Work out the finished part from the listing and answer in its coordinate system (mm). A direction names the side the tool comes from. Coordinates: 2 decimals unless noted, no trailing zeros. Order: outer loops, then holes, each group sorted by start corner. A loop starts at its lowest first (then second) coordinate and runs counter-clockwise, first axis right, second up. Notation, with made-up numbers: (51.5, 78.25) -> (101.5, 78.25) arc R29 ccw to (101.5, 108.25) -> close; hole circle Ø6 at (80, 86.25). An arc over 180 degrees is marked (long way). Use one line per item in the form item = value.
from build123d import *

# Parameters (mm, degrees)
SKETCH1_W           = 1000
SKETCH1_H           = 1000
BOSS_EXTRUDE1_DEPTH = 10
SKETCH2_R           = 150
BOSS_EXTRUDE2_DEPTH = 300
SKETCH3_R           = 25
CUT_EXTRUDE1_DEPTH  = 50


with BuildPart() as part:
    # Sketch1 → Boss-Extrude1 (new body)
    with BuildSketch(Plane(origin=(0, 0, 0), x_dir=(1, 0, 0), z_dir=(0, 1, 0))):
        Rectangle(SKETCH1_W, SKETCH1_H)
    extrude(amount=BOSS_EXTRUDE1_DEPTH)

    # Sketch2 → Boss-Extrude2 (add)
    with BuildSketch(Plane(origin=(0, 10, 0), x_dir=(1, 0, 0), z_dir=(0, 1, 0))):
        with Locations(Location((0, 0, 0), (0, 0, 90))):
            Circle(SKETCH2_R)
    extrude(amount=BOSS_EXTRUDE2_DEPTH)

    # Sketch3 → Cut-Extrude1 (cut)
    with BuildSketch(Plane(origin=(0, 310, 0), x_dir=(1, 0, 0), z_dir=(0, 1, 0))):
        with Locations(Location((0, 0, 0), (0, 0, 270))):
            Circle(SKETCH3_R)
    extrude(amount=-CUT_EXTRUDE1_DEPTH, mode=Mode.SUBTRACT)


solid = part.part
(1) Section A-A on x = 0 is taken. Write down the section's boundary in (y, z), plus the area to 3 significant figures.
Data:
outline = (0, -500) -> (10, -500) -> (10, -150) -> (310, -150) -> (310, -25) -> (260, -25) -> (260, 25) -> (310, 25) -> (310, 150) -> (10, 150) -> (10, 500) -> (0, 500) -> close
area = 97,500 mm²
(2) Section C-C on y = 221 is taken. Write down the section's boundary in (x, z), plus the area to 3 significant figures.
Data:
outline = circle Ø300 at (0, 0)
area = 70,700 mm²
(3) Section D-D on y = 291.5 is taken. Write down the section's boundary in (x, z), plus the area to 3 significant figures.
Data:
outline = circle Ø300 at (0, 0); hole circle Ø50 at (0, 0)
area = 68,700 mm²
(4) Straight lines are drawn through the part: line 1 along X through (y, z) = (275, 0); line 2 along Y through (x, z) = (-113, -275); line 3 along X through (y, z) = (198.5, 1.5). For each, find the intervals that lie inside material, in ascending order.
Data:
line_1 = -150 to -25, 25 to 150
line_2 = 0 to 10
line_3 = -149.99 to 149.99
(5) Section B-B on z = 0 is taken. Write down the section's boundary in (x, y).
Data:
outline = (-500, 0) -> (500, 0) -> (500, 10) -> (150, 10) -> (150, 310) -> (25, 310) -> (25, 260) -> (-25, 260) -> (-25, 310) -> (-150, 310) -> (-150, 10) -> (-500, 10) -> close
(6) The mould has two halves that part along Z. Classify faces 1 (the flat face through (0, 260, 0)), 2 (the flat face through (-118, 10, -118)), 3 (the cylindrical face through (91.273, 157.9, 119.035)): released by +Z, released by -Z, zero draft, split by the parting line, or undercut.
Data:
face_1 = undercut
face_2 = zero draft
face_3 = split by the parting line
(7) Which of the six approach directions +Z, -Z, +X, -X, +Y, -Y give full straight-line access (tool end or side, diameter ignored) to faces 4 (the cylindrical face through (7.509, 285.35, 23.846)), 5 (the flat face through (31, 310, 2))?
Data:
face_4 = +Y
face_5 = +Z, -Z, +X, -X, +Y
(8) Each of these flat-tipped pins is pushed along its axis until it touches: P1, Ø4, axis at y = 69.5, z = 13, coming from the -X side; P2, Ø12, axis at x = 335, z = -256, coming from the +Y side; P3, Ø6, axis at x = 44, y = 135.5, coming from the -Z side. Where does it stop, or does it pass through?
Data:
P1 = -149.6
P2 = 10
P3 = -144.29
